Geometry: final body of the model. Coordinates: model frame, mm. A direction names the side the tool comes from. Give positions to 0.01 mm unless a question says otherwise; leave off trailing zeros. Write each loop counter-clockwise with the first axis right and the second up, starting at its lowest first coordinate (ties: lowest second). Pieces come first, ordered by that corner, then holes. Notation, with made-up numbers: (36, 52) -> (66, 52) arc R24 ccw to (66, 66) -> close; hole circle Ø6 at (6, 58.5). An arc over 180 degrees is marked (long way). Answer as a JSON object with one key per item and string values. Group by question number.
(1) Section query C-C on y = 147. Output: boundary loops of the cut face in (x, z), plus the area to 3 significant figures.
(2) Section query D-D on y = 165.1. Output: boundary loops of the cut face in (x, z), plus the area to 3 significant figures.
(3) Set-up query: faces 1 (the face through (25, 88, -1.587)), 2 (the face through (49.995, 86.408, -13.253)). Return all of +Z, -Z, +X, -X, +Y, -Y with unobstructed straight access to the full face (end or side cutting, diameter ignored); none if empty.
(4) Material intervals for probe 1 along X at (y, z) = (167, -14.75); probe 2 along Z at (x, y) = (1, 114); probe 3 along Z at (x, y) = (24.5, 45.5), sorted ascending.
(5) Draft query along Y for faces 3 (the face through (49.212, 88, -10)), 4 (the face through (23, 177.8, -1)), 5 (the face through (0.783, 111.808, -13.253)). Return one class per face: +Y half, -Y half, draft (parallel to the pull), parting line (faces both ways), or undercut.
(6) Section query A-A on x = 8.5. Output: boundary loops of the cut face in (y, z), plus the area to 3 significant figures.
(7) Section query B-B on z = -7.75. Output: boundary loops of the cut face in (x, y).
from build123d import *

# Parameters (mm, degrees)
SKETCH2_W           = 50.8
SKETCH2_H           = 25.4
SKETCH2_W_2         = 47.625
SKETCH2_H_2         = 22.225
BOSS_EXTRUDE2_DEPTH = 177.8
SKETCH4_R           = 2.5527
CUT_EXTRUDE2_DEPTH  = 50.8
LPATTERN1_COUNT     = 27
LPATTERN1_PITCH     = 6.35
SKETCH5_R           = 2.5527
CUT_EXTRUDE3_DEPTH  = 50.8
LPATTERN2_COUNT     = 5
LPATTERN2_PITCH     = 25.4


with BuildPart() as part:
    # Sketch2 → Boss-Extrude2 (new body)
    with BuildSketch(Plane(origin=(0, 0, 0), x_dir=(1, 0, 0), z_dir=(0, 1, 0))):
        with Locations((25.4, 12.7)):
            Rectangle(SKETCH2_W, SKETCH2_H)
        with Locations((25.4, 12.7)):
            Rectangle(SKETCH2_W_2, SKETCH2_H_2, mode=Mode.SUBTRACT)
    extrude(amount=BOSS_EXTRUDE2_DEPTH)

    # Sketch4 → Cut-Extrude2 (cut)
    with BuildSketch(Plane.ZY):
        with Locations((-12.7, 171.45)):
            Circle(SKETCH4_R)
    cut_extrude2 = extrude(amount=-CUT_EXTRUDE2_DEPTH, mode=Mode.SUBTRACT)

    # LPattern1: Cut-Extrude2 ×27, 21 skipped
    with Locations(*[(0, -i * LPATTERN1_PITCH, 0) for i in range(1, LPATTERN1_COUNT) if i not in (3, 4, 5, 6, 7, 8, 9, 10, 11, 12, 13, 14, 15, 16, 17, 18, 19, 20, 21, 22, 23)]):
        add(cut_extrude2, mode=Mode.SUBTRACT)

    # Sketch5 → Cut-Extrude3 (cut)
    with BuildSketch(Plane.ZY):
        with Locations((-12.7, 139.7)):
            Circle(SKETCH5_R)
    cut_extrude3 = extrude(amount=-CUT_EXTRUDE3_DEPTH, mode=Mode.SUBTRACT)

    # LPattern2: Cut-Extrude3 ×5
    with Locations(*[(0, -i * LPATTERN2_PITCH, 0) for i in range(1, LPATTERN2_COUNT)]):
        add(cut_extrude3, mode=Mode.SUBTRACT)


solid = part.part
Answer list:
{
 "1": {"outline": "(0, -25.4) -> (50.8, -25.4) -> (50.8, 0) -> (0, 0) -> close; hole (1.59, -23.81) -> (49.21, -23.81) -> (49.21, -1.59) -> (1.59, -1.59) -> close", "area": "232 mm2"},
 "2": {"outline": "(0, -25.4) -> (50.8, -25.4) -> (50.8, -15.25) -> (49.21, -15.25) -> (49.21, -23.81) -> (1.59, -23.81) -> (1.59, -15.25) -> (0, -15.25) -> close; (0, -10.15) -> (1.59, -10.15) -> (1.59, -1.59) -> (49.21, -1.59) -> (49.21, -10.15) -> (50.8, -10.15) -> (50.8, 0) -> (0, 0) -> close", "area": "216 mm2"},
 "3": {"face 1": "+Y, -Y", "face 2": "+X, -X"},
 "4": {"probe 1": "0 to 1.59, 49.21 to 50.8", "probe 2": "-25.4 to -15.24, -10.16 to 0", "probe 3": "-25.4 to -23.81, -1.59 to 0"},
 "5": {"face 3": "draft", "face 4": "+Y half", "face 5": "undercut"},
 "6": {"outline": "(0, -25.4) -> (177.8, -25.4) -> (177.8, -23.81) -> (0, -23.81) -> close; (0, -1.59) -> (177.8, -1.59) -> (177.8, 0) -> (0, 0) -> close", "area": "565 mm2"},
 "7": {"outline": "(0, 0) -> (1.59, 0) -> (1.59, 177.8) -> (0, 177.8) -> close; (49.21, 0) -> (50.8, 0) -> (50.8, 177.8) -> (49.21, 177.8) -> close"}
}
